```python
from build123d import *

# Parameters (mm, degrees)
SKETCH_R     = 55
PAD_DEPTH    = 3
PAD001_DEPTH = 8
PAD002_DEPTH = 8
SKETCH003_R  = 1.3
SKETCH003_W  = 3
SKETCH003_H  = 24
POCKET_DEPTH = 5


with BuildPart() as part:
    # Sketch → Pad (new body)
    with BuildSketch(Plane.XY):
        Circle(SKETCH_R)
    extrude(amount=PAD_DEPTH)

    # Sketch001 (on Face3 of Pad) → Pad001 (join)
    with BuildSketch(Plane.XY.offset(3)):
        Polygon((33.500008, 0), (33.500008, 13), (53.345406, 13), (53.345406, 11), (35.5, 11), (35.5, -0.005684), (35.5, -12), (33.500008, -12), align=None)
        Polygon((-33.5, 0), (-33.5, -13), (-53.293575, -13), (-53.293575, -11), (-35.5, -11), (-35.5, 0.001212), (-35.5, 12), (-33.5, 12), align=None)
    extrude(amount=PAD001_DEPTH)

    # Sketch002 (on Face3 of Pad001) → Pad002 (join)
    with BuildSketch(Plane.XY.offset(3)):
        with BuildLine():
            ThreePointArc((-23.973944, -49.5), (-12.298374, -53.607369), (0, -55))
            Line((0, -49.5), (0, -55))
            Line((-23.973944, -49.5), (0, -49.5))
        make_face()
        with BuildLine():
            ThreePointArc((23.973944, 49.5), (12.298374, 53.607369), (0, 55))
            Line((0, 49.5), (0, 55))
            Line((23.973944, 49.5), (0, 49.5))
        make_face()
    extrude(amount=PAD002_DEPTH)

    # Sketch003 (on Face3 of Pad002) → Pocket (cut)
    with BuildSketch(Plane.XY.offset(3)):
        with Locations((-44, -20)):
            Circle(SKETCH003_R)
        with Locations((44, 20)):
            Circle(SKETCH003_R)
        with Locations((32, 0)):
            Rectangle(SKETCH003_W, SKETCH003_H)
        with Locations((-32, 0)):
            Rectangle(SKETCH003_W, SKETCH003_H)
    extrude(amount=-POCKET_DEPTH, mode=Mode.SUBTRACT)


solid = part.part
```
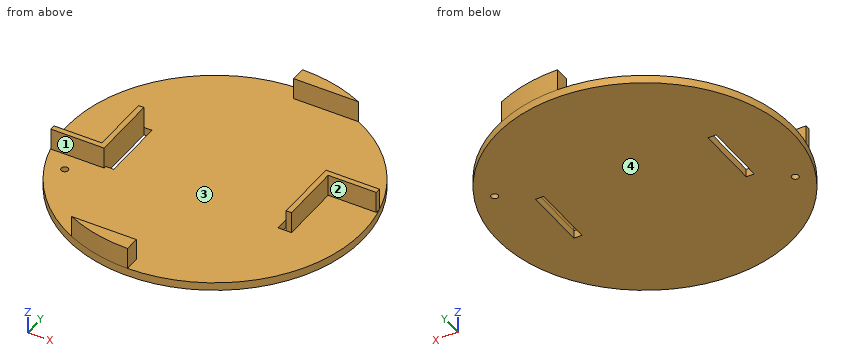
CAD build for the part. Positions are in the model's coordinates, mm. Face numbers are marked on the shaded views. A direction names the side the tool comes from. Coordinates: 2 decimals unless noted, no trailing zeros. Write each loop counter-clockwise with the first axis right and the second up, starting at its lowest first coordinate (ties: lowest second). Pieces come first, ordered by that corner, then holes. Notation, with made-up numbers: (11, 12) -> (22, 12) arc R26 ccw to (22, 43) -> close; hole circle Ø8 at (9.25, -16.5). An arc over 180 degrees is marked (long way). Return JSON: item names as keys, results as strings. Group by question number.
Q1. Cut at D-D, the plane y = -20. Give the cut face in (x, z), then the cut area to 3 significant figures.
Q2. Which spindle directions (+Z, -Z, +X, -X, +Y, -Y) get a long thin tool onto all of the face, cutting with end or side? Do the marked faces 1 and 2. Say none if no direction does.
Q3. Drill centre lines: line 1 (X direction, y = -3.5, z = 6); line 2 (Z direction, x = 17, y = -44); line 3 (Y direction, x = 43, z = 9.5). Where is each one in solid material? Low to high.
Q4. Flat gauge pins, fed straight in: pin 1 (5.5 mm diameter, centred on y = -1.5, z = 6.5, fed in from +X); pin 2 (1.5 mm diameter, centred on x = 31.5, z = 2, fed in from +Y); pin 3 (2.5 mm diameter, centred on x = 44.5, z = 8, fed in from -Y); pin 4 (3 mm diameter, centred on x = 25, y = -25, fed in from -Z). Where does each tip first touch, or does it go through?
Q5. Cut at C-C, the plane z = 7. Give the cut face in (x, y).
Q6. Cut at A-A, the plane x = 44. Give the cut face in (y, z), then the cut area to 3 significant figures.
Q7. Pull direction X, two halves, no side cores. Call the marked faces 3 and 4: released by +X, released by -X, zero draft, split by the parting line, or undercut.
Q8. Cut at B-B, the plane y = 0. State how many separate pieces and enclosed holes the cut face has, then the cut area to 3 significant figures.
Returned:
{
 "1": {"outline": "(-51.23, 0) -> (-45.3, 0) -> (-45.3, 3) -> (-51.23, 3) -> close; (-42.7, 0) -> (51.23, 0) -> (51.23, 3) -> (-42.7, 3) -> close", "area": "300 mm2"},
 "2": {"face 1": "+Z, +X, -X, -Y", "face 2": "+Z, +X, -Y"},
 "3": {"line 1": "x = -35.5 to -33.5, 33.5 to 35.5", "line 2": "z = 0 to 3", "line 3": "y = 11 to 13"},
 "4": {"pin 1": "stops at x = 35.5", "pin 2": "stops at y = 45.6", "pin 3": "stops at y = 11", "pin 4": "stops at z = 0"},
 "5": {"outline": "(-53.29, -13) -> (-33.5, -13) -> (-33.5, 12) -> (-35.5, 12) -> (-35.5, -11) -> (-53.29, -11) -> close; (-23.97, -49.5) arc R55 ccw to (0, -55) -> (0, -49.5) -> close; (0, 49.5) -> (23.97, 49.5) arc R55 ccw to (0, 55) -> close; (33.5, -12) -> (35.5, -12) -> (35.5, 11) -> (53.35, 11) -> (53.35, 13) -> (33.5, 13) -> close"},
 "6": {"outline": "(-33, 0) -> (18.7, 0) -> (18.7, 3) -> (13, 3) -> (13, 11) -> (11, 11) -> (11, 3) -> (-33, 3) -> close; (21.3, 0) -> (33, 0) -> (33, 3) -> (21.3, 3) -> close", "area": "206 mm2"},
 "7": {"face 3": "undercut", "face 4": "zero draft"},
 "8": {"separate pieces": "3", "enclosed holes": "0", "area": "344 mm2"}
}
